from build123d import *

# Parameters (mm, degrees)
SKETCH_1_R          = 32.5
SKETCH_1_R_2        = 5
EXTRUDE_1_DEPTH     = 9
SKETCH_2_R          = 10
CUT_EXTRUDE_2_DEPTH = 15
CUT_EXTRUDE_3_DEPTH = 45
FILLET_1_R          = 1.5


with BuildPart() as part:
    # 草图1 → 凸台-拉伸1 (new, symmetric)
    with BuildSketch(Plane.XY):
        Circle(SKETCH_1_R)
        Circle(SKETCH_1_R_2, mode=Mode.SUBTRACT)
    extrude(amount=EXTRUDE_1_DEPTH, both=True)

    # 草图2 → 切除-拉伸2 (cut)
    with BuildSketch(Plane.XY.offset(9)):
        Circle(SKETCH_2_R)
    extrude(amount=-CUT_EXTRUDE_2_DEPTH, mode=Mode.SUBTRACT)

    # 草图3 → 切除-拉伸3 (cut)
    with BuildSketch(Plane.XY.offset(9)):
        with BuildLine():
            ThreePointArc((-13.460032078, 8.65029112), (-11.886088914, 10.710783834), (-10, 12.489995997))
            Line((-10, 12.489995997), (6.490409144, 25.692889856))
            ThreePointArc((6.490409144, 25.692889856), (-4.927079416, 26.037931723), (-15.429116278, 21.545124063))
            Line((-15.429116278, 21.545124063), (-13.460032078, 8.65029112))
        make_face()
        with BuildLine():
            ThreePointArc((25.495899884, 7.225585728), (20.085970626, 17.285941802), (10.944066627, 24.134568686))
            Line((10.944066627, 24.134568686), (0.761355821, 15.981875275))
            ThreePointArc((0.761355821, 15.981875275), (3.332766438, 15.649046868), (5.816653826, 14.905252036))
            Line((5.816653826, 14.905252036), (25.495899884, 7.225585728))
        make_face()
        with BuildLine():
            ThreePointArc((26.5, 0), (26.468276738, 1.296274087), (26.373182905, 2.589444623))
            Line((26.373182905, 2.589444623), (14.221387899, 7.331584155))
            ThreePointArc((14.221387899, 7.331584155), (15.218855351, 4.938263034), (15.816653826, 2.415256039))
            Line((15.816653826, 2.415256039), (19.005490739, -18.467304128))
            ThreePointArc((19.005490739, -18.467304128), (24.554994447, -9.965051315), (26.5, 0))
        make_face()
        with BuildLine():
            Line((15.429116278, -21.545124063), (13.460032078, -8.65029112))
            ThreePointArc((13.460032078, -8.65029112), (11.886088914, -10.710783834), (10, -12.489995997))
            Line((10, -12.489995997), (-6.490409144, -25.692889856))
            ThreePointArc((-6.490409144, -25.692889856), (4.927079416, -26.037931723), (15.429116278, -21.545124063))
        make_face()
        with BuildLine():
            Line((-5.816653826, -14.905252036), (-25.495899884, -7.225585728))
            ThreePointArc((-25.495899884, -7.225585728), (-20.085970626, -17.285941802), (-10.944066627, -24.134568686))
            Line((-10.944066627, -24.134568686), (-0.761355821, -15.981875275))
            ThreePointArc((-0.761355821, -15.981875275), (-3.332766438, -15.649046868), (-5.816653826, -14.905252036))
        make_face()
        with BuildLine():
            Line((-15.816653826, -2.415256039), (-19.005490739, 18.467304128))
            ThreePointArc((-19.005490739, 18.467304128), (-25.013050042, 8.751989921), (-26.373182905, -2.589444623))
            Line((-26.373182905, -2.589444623), (-14.221387899, -7.331584155))
            ThreePointArc((-14.221387899, -7.331584155), (-15.218855351, -4.938263034), (-15.816653826, -2.415256039))
        make_face()
    extrude(amount=-CUT_EXTRUDE_3_DEPTH, mode=Mode.SUBTRACT)

    # 圆角1
    fillet_1_edges = [part.edges().sort_by_distance(p)[0] for p in [
        (-6.490409144, -25.692889856, 0),
        (13.460032078, -8.65029112, 0),
        (15.429116278, -21.545124063, 0),
        (-25.495899884, -7.225585728, 0),
        (-0.761355821, -15.981875275, 0),
        (-10.944066627, -24.134568686, 0),
        (25.495899884, 7.225585728, 0),
        (0.761355821, 15.981875275, 0),
        (10.944066627, 24.134568686, 0),
        (19.005490739, -18.467304128, 0),
        (14.221387899, 7.331584155, 0),
        (26.373182905, 2.589444623, 0),
        (-19.005490739, 18.467304128, 0),
        (-14.221387899, -7.331584155, 0),
        (-26.373182905, -2.589444623, 0),
        (6.490409144, 25.692889856, 0),
        (-13.460032078, 8.65029112, 0),
        (-15.429116278, 21.545124063, 0),
    ]]
    fillet(fillet_1_edges, radius=FILLET_1_R)


solid = part.part
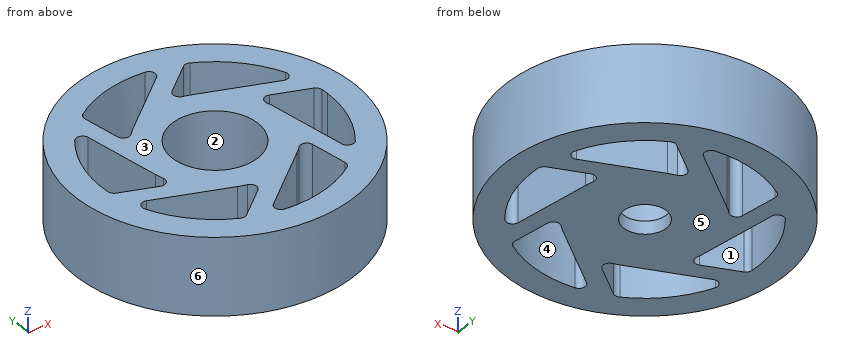
Can you work these out from the model? Positions are in its coordinate system, mm. Face numbers are marked on the shaded views. A direction names the side the tool comes from. Coordinates: 2 decimals unless noted, no trailing zeros. Loops run counter-clockwise (first coordinate to the right, second up) from the corner with the lowest first, then second, coordinate; pieces in that order, holes last. Notation, with made-up numbers: (87.25, 1.5) - (93.25, 1.5) arc R8 cw to (93.25, 8.5) - close; hole circle Ø3 at (25.5, 58). An arc over 180 degrees is marked (long way). Put each result on its own line as item: value. Start each with the question number.
Item 1: Suppose I cut it at D-D (y = 28). Please give me the cut outline in (x, z).
Item 2: For pin 1 (2 mm diameter, centred on x = 10.5, z = -6.5, fed in from +Y); pin 2 (6 mm diameter, centred on x = 24.5, z = -0.5, fed in from -Y); pin 3 (4 mm diameter, centred on y = 18.5, z = 1, fed in from +X); pin 4 (4 mm diameter, centred on x = 16.5, y = 13.5, fed in from -Z), each with a flat end and sliding along its axis, tell me the tip position at first contact or that it passes through.
Item 3: If I drill on line 1 along Y through (x, z) = (-0.5, 2); line 2 along Y through (x, z) = (0, -8.05); line 3 along X through (y, z) = (22, 7.5), over which ranges is the centre line in solid material (lowest first)?
Item 4: Suppose I cut it at C-C (z = 2.75). State how many separate pieces and enclosed holes the cut face has, and give its area (3 significant figures).
Item 5: Which directions (+Z, -Z, +X, -X, +Y, -Y) give clear straight access to the entire face, cutting with the end or side of a thin tool? Please do the marked faces 1, 2 and 3.
Item 6: Suppose I cut it at B-B (x = 0). Please give me the cut outline in (y, z).
Item 7: Suppose I cut it at A-A (y = 19.5). Please give me the cut outline in (x, z), and give its area (3 significant figures).
Item 8: If we mould it in two halves opening along X, with no side actions, what happens to the marked faces 4, 5 and 6? For each: +X half, -X half, draft (parallel to the pull), parting line (faces both ways), or undercut.
Here are the results:
1. outline: (-16.5, -9) - (16.5, -9) - (16.5, 9) - (-16.5, 9) - close
2. pin 1: y = 31.08
2. pin 2: y = -24.37
2. pin 3: x = 28
2. pin 4: through
3. line 1: -32.5 to -26.5, -20.9 to -9.99, 9.99 to 20.1, 26.5 to 32.5
3. line 2: -32.5 to -26.5, -20.5 to -5, 5 to 20.5, 26.5 to 32.5
3. line 3: -23.92 to -14.76, 1.88 to 8.28, 14.77 to 23.92
4. separate pieces: 1
4. enclosed holes: 7
4. area: 2,000 mm²
5. face 1: +Z, -Z
5. face 2: +Z
5. face 3: +Z, +X, -X, +Y, -Y
6. outline: (-32.5, -9) - (-26.5, -9) - (-26.5, 9) - (-32.5, 9) - close; (-20.5, -9) - (-5, -9) - (-5, -6) - (-10, -6) - (-10, 9) - (-20.5, 9) - close; (5, -9) - (20.5, -9) - (20.5, 9) - (10, 9) - (10, -6) - (5, -6) - close; (26.5, -9) - (32.5, -9) - (32.5, 9) - (26.5, 9) - close
7. outline: (-26, -9) - (-15.12, -9) - (-15.12, 9) - (-26, 9) - close; (-1.24, -9) - (5.16, -9) - (5.16, 9) - (-1.24, 9) - close; (17.94, -9) - (26, -9) - (26, 9) - (17.94, 9) - close
7. area: 456 mm²
8. face 4: undercut
8. face 5: draft
8. face 6: parting line
